Source: CAD feature listing. Evaluate the final solid. Frame: model axes, mm. Face numbers are marked on the shaded views. A direction names the side the tool comes from. Round coordinates to 2 decimals unless told otherwise and drop trailing zeros. Write each loop counter-clockwise with the first axis right and the second up, starting at its lowest first coordinate (ties: lowest second). Pieces come first, ordered by that corner, then holes. Notation, with made-up numbers: M 52.5,89 L 110.5,89 A19 ccw 110.5,108 Z; hole C 85,38 d7. An arc over 180 degrees is marked long. Answer in a Markdown table with one row per item.
from build123d import *

# Parameters (mm, degrees)
F1_DEPTH = 25
F2_R     = 2.75
F2_R_2   = 1.75
F3_DEPTH = 50
F4_R     = 11
F5_R     = 10
F6_R     = 2.5
F7_R     = 3


with BuildPart() as f1:
    # F0 (on Top) → F1 (new body)
    with BuildSketch(Plane.XY):
        with BuildLine():
            ThreePointArc((2.5, -12.539936204), (0, -12.7867118525), (-2.5, -12.539936204))
            Line((-2.5, -12.539936204), (-2.5, -32.0420756284))
            Line((-2.5, -32.0420756284), (0, -32.0420756284))
            Line((0, -32.0420756284), (2.5, -32.0420756284))
            Line((2.5, -32.0420756284), (2.5, -12.539936204))
        make_face()
        with BuildLine():
            ThreePointArc((-6.0296314677, 11.2757946223), (-4.0714568053, 12.1211896892), (-2, 12.6293309403))
            Line((-2, 12.6293309403), (-2, 20.9377203137))
            Line((-2, 20.9377203137), (-6.0296314677, 20.9377203137))
            Line((-6.0296314677, 20.9377203137), (-6.0296314677, 11.2757946223))
        make_face()
        with BuildLine():
            ThreePointArc((-6.0296314677, 8.5961354319), (-4.1050168721, 9.6643073461), (-2, 10.307764064))
            Line((-2, 10.307764064), (-2, 12.6293309403))
            ThreePointArc((-2, 12.6293309403), (-4.0714568053, 12.1211896892), (-6.0296314677, 11.2757946223))
            Line((-6.0296314677, 11.2757946223), (-6.0296314677, 8.5961354319))
        make_face()
        with BuildLine():
            ThreePointArc((2, 10.307764064), (4.1050168721, 9.6643073461), (6.0296314677, 8.5961354319))
            Line((6.0296314677, 8.5961354319), (6.0296314677, 11.2757946223))
            ThreePointArc((6.0296314677, 11.2757946223), (4.0714568053, 12.1211896892), (2, 12.6293309403))
            Line((2, 12.6293309403), (2, 10.307764064))
        make_face()
        with BuildLine():
            ThreePointArc((2, 12.6293309403), (4.0714568053, 12.1211896892), (6.0296314677, 11.2757946223))
            Line((6.0296314677, 11.2757946223), (6.0296314677, 20.9377203137))
            Line((6.0296314677, 20.9377203137), (2, 20.9377203137))
            Line((2, 20.9377203137), (2, 13.3510299228))
            Line((2, 13.3510299228), (2, 12.6293309403))
        make_face()
        with BuildLine():
            ThreePointArc((6.0296314677, 8.5961354319), (0, -10.5), (-6.0296314677, 8.5961354319))
            Line((-6.0296314677, 8.5961354319), (-6.0296314677, 11.2757946223))
            ThreePointArc((-6.0296314677, 11.2757946223), (-12.648553749, -1.8745901043), (-2.5, -12.539936204))
            ThreePointArc((-2.5, -12.539936204), (0, -12.7867118525), (2.5, -12.539936204))
            ThreePointArc((2.5, -12.539936204), (12.648553749, -1.8745901043), (6.0296314677, 11.2757946223))
            Line((6.0296314677, 11.2757946223), (6.0296314677, 8.5961354319))
        make_face()
    extrude(amount=F1_DEPTH)

    # F2 (on face) → F3 (cut)
    with BuildSketch(Plane(origin=(-6.0296314677, 0, 0), x_dir=(0, -1, 0), z_dir=(-1, 0, 0))):
        with Locations((24.539936204, 12.5)):
            Circle(F2_R)
        with Locations((-17.6877203137, 12.5)):
            Circle(F2_R_2)
    extrude(amount=-F3_DEPTH, mode=Mode.SUBTRACT)

    # F4
    f4_edges = [f1.edges().sort_by_distance(p)[0] for p in [
        (0, -32.042076, 25),
    ]]
    fillet(f4_edges, radius=F4_R)

    # F5
    f5_edges = [f1.edges().sort_by_distance(p)[0] for p in [
        (0, -32.042076, 0),
    ]]
    fillet(f5_edges, radius=F5_R)

    # F6
    f6_edges = [f1.edges().sort_by_distance(p)[0] for p in [
        (-4.014816, 20.93772, 25),
        (4.014816, 20.93772, 25),
        (4.014816, 20.93772, 0),
        (-4.014816, 20.93772, 0),
    ]]
    fillet(f6_edges, radius=F6_R)

    # F7
    f7_edges = [f1.edges().sort_by_distance(p)[0] for p in [
        (-2, 10.307764, 12.5),
        (2, 10.307764, 12.5),
    ]]
    fillet(f7_edges, radius=F7_R)


solid = f1.part
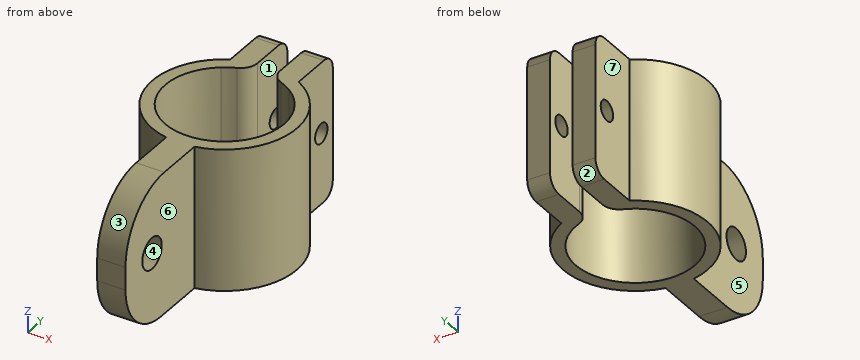
Q1. Pull-direction query (Z, two-part tool) for the marked faces 1, 2, 3 and 4; classes: pulls with the +Z half, pulls with the -Z half, needs draft (parallel to the pull), parting line crosses it, or undercut.
Solutions:
| item | result |
|---|---|
| face 1 | needs draft |
| face 2 | pulls with the -Z half |
| face 3 | pulls with the +Z half |
| face 4 | undercut |
Q2. Material intervals for probe 1 along X at (y, z) = (16.5, 17.75); probe 2 along X at (y, z) = (0.5, 22.75); probe 3 along Y at (x, z) = (-4.5, 11.5), sorted ascending.
Solutions:
| item | result |
|---|---|
| probe 1 | x = -6.03 to -2, 2 to 6.03 |
| probe 2 | x = -12.78 to -10.49, 10.49 to 12.78 |
| probe 3 | y = -11.97 to -9.49, 9.49 to 16.25, 19.12 to 20.94 |
Q3. Section B-B (y = 0). Return loops of the section in (x, z).
Solutions:
| item | result |
|---|---|
| outline | M -12.79,0 L -10.5,0 L -10.5,25 L -12.79,25 Z; M 10.5,0 L 12.79,0 L 12.79,25 L 10.5,25 Z |
Q4. Section A-A (z = 12.5). Return loops of the section in (x, y).
Solutions:
| item | result |
|---|---|
| outline | M -6.03,11.28 A12.79 ccw -2.5,-12.54 L -2.5,-21.79 L 2.5,-21.79 L 2.5,-12.54 A12.79 ccw 6.03,11.28 L 6.03,15.94 L 2,15.94 L 2,12.54 A3 ccw 3.89,9.75 A10.5 cw long -3.89,9.75 A3 ccw -2,12.54 L -2,15.94 L -6.03,15.94 Z; M -6.03,19.44 L -2,19.44 L -2,20.94 L -6.03,20.94 Z; M -2.5,-32.04 L 2.5,-32.04 L 2.5,-27.29 L -2.5,-27.29 Z; M 2,19.44 L 6.03,19.44 L 6.03,20.94 L 2,20.94 Z |
Q5. Section C-C (x = 0.75). Return loops of the section in (y, z).
Solutions:
| item | result |
|---|---|
| outline | M -32.04,10 A10 ccw -22.04,0 L -10.47,0 L -10.47,25 L -21.04,25 A11 ccw -32.04,14 Z; hole C -24.54,12.5 d5.5 |
Q6. Section D-D (z = 4.75). Return loops of the section in (x, y).
Solutions:
| item | result |
|---|---|
| outline | M -6.03,11.28 A12.79 ccw -2.5,-12.54 L -2.5,-30.55 L 2.5,-30.55 L 2.5,-12.54 A12.79 ccw 6.03,11.28 L 6.03,20.94 L 2,20.94 L 2,12.54 A3 ccw 3.89,9.75 A10.5 cw long -3.89,9.75 A3 ccw -2,12.54 L -2,20.94 L -6.03,20.94 Z |
Q7. Access query for the marked faces 5, 6 and 7. Directions: +Z, -Z, +X, -X, +Y, -Y. A direction counts if a zero-diameter tool reaches every point of the face in a straight line with its end or side. Return the directions, or none.
Solutions:
| item | result |
|---|---|
| face 5 | +Z, -Z, -X, -Y |
| face 6 | +Z, -Z, +X, -Y |
| face 7 | +Z, -Z, -X, +Y |
Q8. Contact query for flat-ended pins moving along their axis: pin 1 Ø2 at (x, z) = (10, 3.5) entering from -Y; pin 2 Ø10 at (y, z) = (-25, 18) entering from -X; pin 3 Ø5.5 at (y, z) = (17.69, 12.5) entering from +X. Output: stop coordinate, or through.
Solutions:
| item | result |
|---|---|
| pin 1 | stops at y = -9.08 |
| pin 2 | stops at x = -2.5 |
| pin 3 | stops at x = 6.03 |
